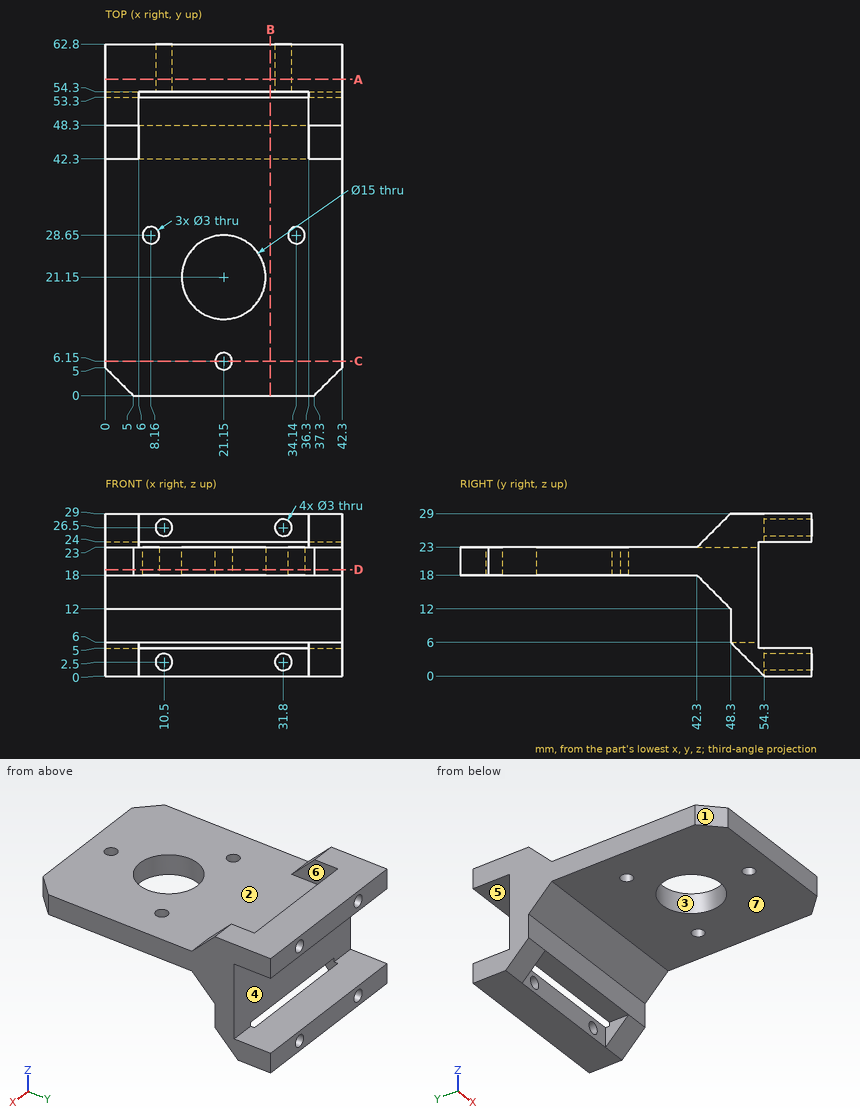
Design review of the part shown in the three views and the two pictorial views. Dimensions are in mm from the part's minimum x, y and z. A direction names the side the tool comes from. Round coordinates to 2 decimals unless told otherwise and drop trailing zeros. Write each loop counter-clockwise with the first axis right and the second up, starting at its lowest first coordinate (ties: lowest second). Pieces come first, ordered by that corner, then holes.
1) Mouldability with a two-part tool opening along Y and no side actions: class the marked faces 1, 2, 3 and 4 as +Y half, -Y half, draft (parallel to the pull), parting line (faces both ways), or undercut.
Answer below:
face 1: -Y half
face 2: draft
face 3: undercut
face 4: +Y half
2) Machinability: for the marked faces 5, 6 and 7, which of the approach directions +Z, -Z, +X, -X, +Y, -Y give a long, thin tool a straight path to every point of the face, cutting with its end or side? Answer none if there is none.
Answer below:
face 5: +X, -X, +Y
face 6: +Z, -Y
face 7: -Z, +X, -X, -Y
3) Take a section at B-B on x = 29.5. State how many separate pieces and enclosed holes the cut face has.
Answer below:
separate pieces: 3
enclosed holes: 0
4) Take a section at A-A on y = 56.5. Give the boundary of the cut face in (x, z).
Answer below:
outline: (0, 0) - (42.3, 0) - (42.3, 5) - (0, 5) - close; (0, 24) - (42.3, 24) - (42.3, 29) - (0, 29) - close; hole circle Ø3 at (10.5, 2.5); hole circle Ø3 at (10.5, 26.5); hole circle Ø3 at (31.8, 2.5); hole circle Ø3 at (31.8, 26.5)
5) Take a section at D-D on z = 19. Give the boundary of the cut face in (x, y), then the cut area to 3 significant figures.
Answer below:
outline: (0, 5) - (5, 0) - (37.3, 0) - (42.3, 5) - (42.3, 53.3) - (0, 53.3) - close; hole circle Ø3 at (8.16, 28.65); hole circle Ø15 at (21.15, 21.15); hole circle Ø3 at (21.15, 6.15); hole circle Ø3 at (34.14, 28.65)
area: 2,030 mm2
6) Insertion check: pin 1 Ø2 at (x, z) = (10, 8) entering from +Y; pin 2 Ø3.5 at (x, y) = (21.15, 6.15) entering from +Z; pin 3 Ø4 at (x, y) = (16.5, 50.5) entering from -Z; pin 4 Ø1 at (x, y) = (25.5, 18) entering from +Z. Each pin has a flat end and moves straight along its axis. Give the tip position at first contact, or say it passes through.
Answer below:
pin 1: stops at y = 53.3
pin 2: stops at z = 23
pin 3: stops at z = 6
pin 4: passes through
7) Take a section at C-C on y = 6.15. Give the boundary of the cut face in (x, z).
Answer below:
outline: (0, 18) - (19.65, 18) - (19.65, 23) - (0, 23) - close; (22.65, 18) - (42.3, 18) - (42.3, 23) - (22.65, 23) - close
8) For line 1 along Z through (x, y) = (10.5, 58); line 2 along Y through (x, z) = (21.15, 19.15); line 3 along Z through (x, y) = (10, 58) (1 decimal), list the stretches that pass through material, from the lowest coordinate up.
Answer below:
line 1: z = 0 to 1, 4 to 5, 24 to 25, 28 to 29
line 2: y = 0 to 4.65, 7.65 to 13.65, 28.65 to 53.3
line 3: z = 0 to 1.1, 3.9 to 5, 24 to 25.1, 27.9 to 29
